Can you work these out from the model? Positions are in its coordinate system, mm. Face numbers are marked on the shaded views. A direction names the side the tool comes from. Coordinates: 2 decimals unless noted, no trailing zeros. Write each loop counter-clockwise with the first axis right and the second up, starting at its lowest first coordinate (ties: lowest second). Pieces come first, ordered by that corner, then holes. Notation, with made-up numbers: (71, 65) - (117, 65) arc R25 cw to (117, 90) - close; hole circle Ø9 at (-32.5, 14.5). An arc over 180 degrees is marked (long way). Use one line per item in the form item = value. Start each with the question number.
(1) If we section it at A-A on y = -20: Please give me the cut outline in (x, z).
(2) If I drill on probe 1 along Z at (x, y) = (-14.5, -21); probe 2 along X at (y, z) = (-9.25, 18); probe 3 along Y at (x, z) = (-15, -32), over which ranges is the centre line in solid material (lowest first)? Write a range as from..to.
(3) Thinking about a two-plate mould opening in X: for the marked faces 3, 4 and 5, which applies, pulls with the +X half, pulls with the -X half, needs draft (parallel to the pull), parting line crosses it, or undercut?
(4) On a 3-axis mill with a long thin cutter (end or side, diameter ignored), from which of +Z, -Z, +X, -X, +Y, -Y can I reach the whole of each face in a straight line? I mean the marked faces 1 and 2. Say none if no direction works.
(5) If we section it at D-D on z = 1: Please give me the cut outline in (x, y), then the cut area to 3 significant figures.
(6) If we section it at C-C on y = -10.75: Please give me the cut outline in (x, z).
(7) For pin 1 Ø8 at (x, z) = (-10, 32.5) entering from -Y, with a flat end and sliding along its axis, tell me the tip position at first contact or that it passes through.
(8) If we section it at B-B on x = -8.5: Please give me the cut outline in (y, z).
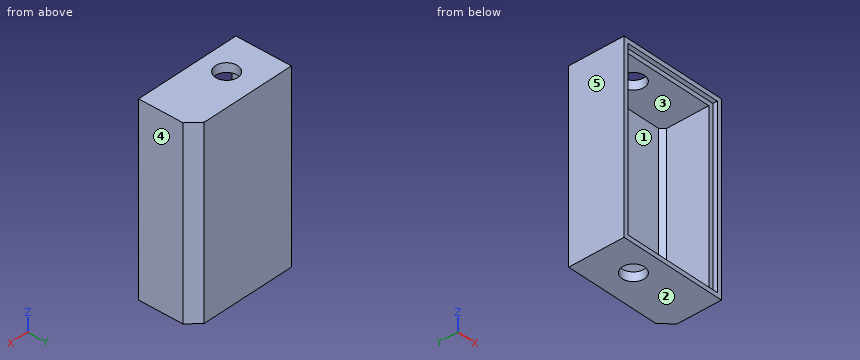
```python
from build123d import *

# Parameters (mm, degrees)
F0_W     = 48
F0_H     = 83
F0_W_2   = 44
F0_H_2   = 79
F0_W_3   = 40
F0_H_3   = 75
F1_DEPTH = 2
F2_DEPTH = 25
F3_DEPTH = 23
F4_SIZE2 = 5
F4_SIZE  = 5
F6_DEPTH = 2
F12_D    = 10


with BuildPart() as f1:
    # F0 (on Front) → F1 (new body)
    with BuildSketch(Plane.XZ):
        Rectangle(F0_W, F0_H)
        Rectangle(F0_W_2, F0_H_2, mode=Mode.SUBTRACT)
        Rectangle(F0_W_2, F0_H_2)
        Rectangle(F0_W_3, F0_H_3, mode=Mode.SUBTRACT)
        Rectangle(F0_W_3, F0_H_3)
    extrude(amount=F1_DEPTH)

    # F0 (on Front) → F2 (join)
    with BuildSketch(Plane.XZ):
        Rectangle(F0_W, F0_H)
        Rectangle(F0_W_2, F0_H_2, mode=Mode.SUBTRACT)
    extrude(amount=F2_DEPTH)

    # F0 (on Front) → F3 (join)
    with BuildSketch(Plane.XZ):
        Rectangle(F0_W_2, F0_H_2)
        Rectangle(F0_W_3, F0_H_3, mode=Mode.SUBTRACT)
    extrude(amount=F3_DEPTH)

    # F4
    f4_edges = [f1.edges().sort_by_distance(p)[0] for p in [
        (24, 0, 0),
    ]]
    chamfer(f4_edges, length=F4_SIZE, length2=F4_SIZE2)

    # F6 (add): a face of the model
    f6_faces = [f1.faces().sort_by_distance(p)[0] for p in [
        (21.5, -2.5, 0),
    ]]
    extrude(f6_faces, amount=-F6_DEPTH)

    # F12 (through all)
    with Locations(Plane.XY.offset(41.5)):
        with Locations((-7.1147754788, -13.7537298724)):
            Hole(F12_D / 2)


solid = f1.part
```
Reported:
q1.outline = (-24, -41.5) - (24, -41.5) - (24, 41.5) - (-24, 41.5) - close; hole (-20, -37.5) - (20, -37.5) - (20, 37.5) - (-20, 37.5) - close
q2.probe_1 = -41.5..-37.5, 37.5..41.5
q2.probe_2 = -24..-20, 20..24
q2.probe_3 = -2..0
q3.face_3 = undercut
q3.face_4 = pulls with the +X half
q3.face_5 = pulls with the -X half
q4.face_1 = -Y
q4.face_2 = -Z, +X, -X, +Y, -Y
q5.outline = (-24, -25) - (-22, -25) - (-22, -23) - (-20, -23) - (-20, -2) - (18.17, -2) - (20, -3.83) - (20, -23) - (22, -23) - (22, -25) - (24, -25) - (24, -5) - (19, 0) - (-24, 0) - close
q5.area = 261 mm2
q6.outline = (-24, -41.5) - (-11.11, -41.5) - (-11.11, -37.5) - (-20, -37.5) - (-20, 37.5) - (-11.11, 37.5) - (-11.11, 41.5) - (-24, 41.5) - close; (-3.12, -41.5) - (24, -41.5) - (24, 41.5) - (-3.12, 41.5) - (-3.12, 37.5) - (20, 37.5) - (20, -37.5) - (-3.12, -37.5) - close
q7.pin_1 = -2
q8.outline = (-25, -41.5) - (-18.56, -41.5) - (-18.56, -37.5) - (-23, -37.5) - (-23, -39.5) - (-25, -39.5) - close; (-25, 39.5) - (-23, 39.5) - (-23, 37.5) - (-18.56, 37.5) - (-18.56, 41.5) - (-25, 41.5) - close; (-8.95, -41.5) - (0, -41.5) - (0, 41.5) - (-8.95, 41.5) - (-8.95, 37.5) - (-2, 37.5) - (-2, -37.5) - (-8.95, -37.5) - close
